Here's the drawing with two shaded views (mm, measured from the low corner). I have some questions. A direction names the side the tool comes from. Round coordinates to 2 decimals unless told otherwise and drop trailing zeros. Loops run counter-clockwise (first coordinate to the right, second up) from the corner with the lowest first, then second, coordinate; pieces in that order, holes last. Notation, with made-up numbers: (65.5, 50.5) -> (115.5, 50.5) arc R20 cw to (115.5, 65.5) -> close; hole circle Ø3 at (-23, 13). An arc over 180 degrees is marked (long way). Use a Markdown table: item, result.
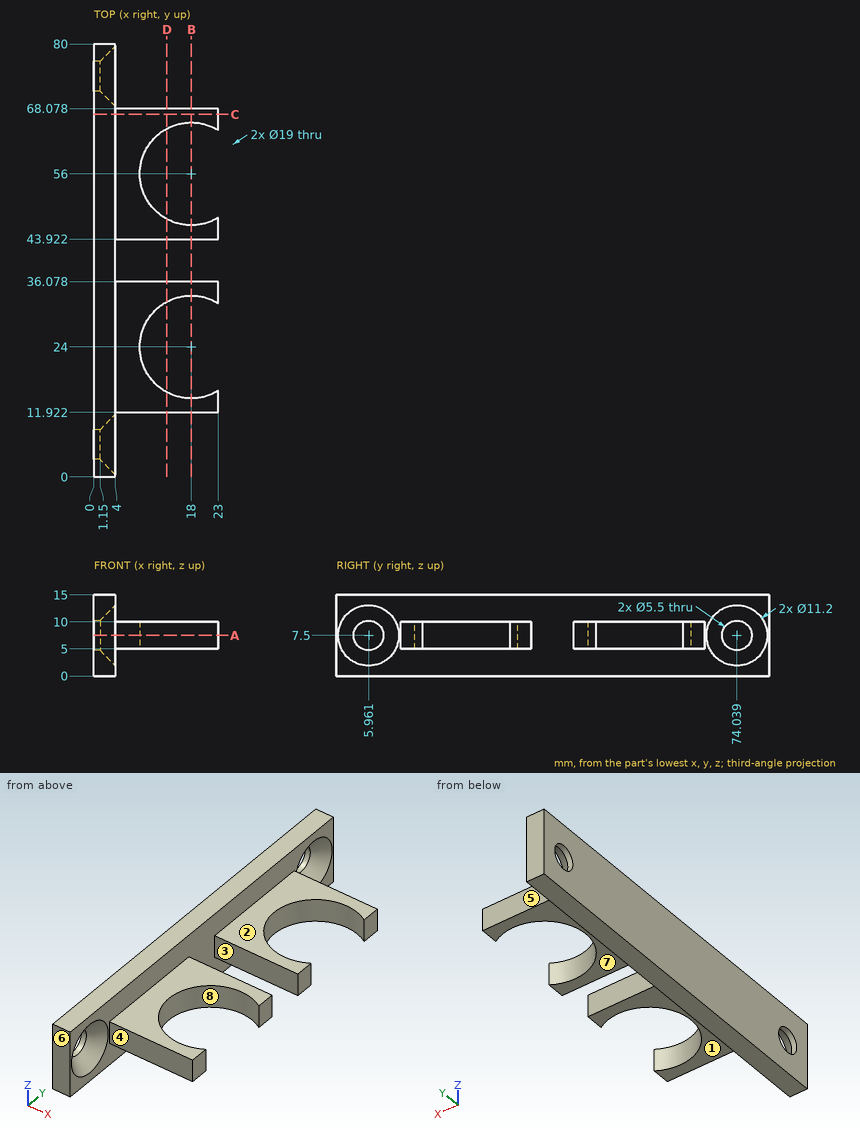
1. I want a section at D-D (x = 13.5). Please give me the cut outline in (y, z).
Answer sheet:
| item | result |
|---|---|
| outline | (11.92, 5) -> (15.63, 5) -> (15.63, 10) -> (11.92, 10) -> close; (32.37, 5) -> (36.08, 5) -> (36.08, 10) -> (32.37, 10) -> close; (43.92, 5) -> (47.63, 5) -> (47.63, 10) -> (43.92, 10) -> close; (64.37, 5) -> (68.08, 5) -> (68.08, 10) -> (64.37, 10) -> close |
2. Which directions (+Z, -Z, +X, -X, +Y, -Y) give clear straight access to the entire face, cutting with the end or side of a thin tool? Please do the marked faces 1, 2, 3, 4 and 5.
Answer sheet:
| item | result |
|---|---|
| face 1 | -Z, +X, +Y, -Y |
| face 2 | +Z, +X, +Y, -Y |
| face 3 | +Z, -Z, +X |
| face 4 | +Z, -Z, +X, -Y |
| face 5 | +Z, -Z, +X, +Y |
3. I want a section at B-B (x = 18). Please give me the cut outline in (y, z).
Answer sheet:
| item | result |
|---|---|
| outline | (11.92, 5) -> (14.5, 5) -> (14.5, 10) -> (11.92, 10) -> close; (33.5, 5) -> (36.08, 5) -> (36.08, 10) -> (33.5, 10) -> close; (43.92, 5) -> (46.5, 5) -> (46.5, 10) -> (43.92, 10) -> close; (65.5, 5) -> (68.08, 5) -> (68.08, 10) -> (65.5, 10) -> close |
4. I need wall thicknesses on line 1 (Y direction, x = 18, z = 6.5); line 2 (Y direction, x = 0.45, z = 7.5); line 3 (Y direction, x = 6.25, z = 8.25). Which ranges of each line are inside material? Lowest first, please.
Answer sheet:
| item | result |
|---|---|
| line 1 | y = 11.92 to 14.5, 33.5 to 36.08, 43.92 to 46.5, 65.5 to 68.08 |
| line 2 | y = 0 to 3.21, 8.71 to 71.29, 76.79 to 80 |
| line 3 | y = 11.92 to 36.08, 43.92 to 68.08 |
5. If we mould it in two halves opening along Y, with no side actions, what happens to the marked faces 6, 7 and 8? For each: +Y half, -Y half, draft (parallel to the pull), parting line (faces both ways), or undercut.
Answer sheet:
| item | result |
|---|---|
| face 6 | -Y half |
| face 7 | draft |
| face 8 | undercut |
6. Will these pins go through, and if not, where does the flat tip stop? pin 1 Ø6 at (y, z) = (38, 12) entering from +X; pin 2 Ø8 at (x, z) = (15.5, 8.5) entering from -Y; pin 3 Ø6 at (x, y) = (10.5, 50.5) entering from -Z; pin 4 Ø9.5 at (x, y) = (14.5, 29.5) entering from +Z.
Answer sheet:
| item | result |
|---|---|
| pin 1 | stops at x = 23 |
| pin 2 | stops at y = 11.92 |
| pin 3 | stops at z = 5 |
| pin 4 | stops at z = 10 |
7. I want a section at C-C (y = 67). Please give me the cut outline in (x, z), plus the area to 3 significant figures.
Answer sheet:
| item | result |
|---|---|
| outline | (0, 0) -> (4, 0) -> (4, 5) -> (23, 5) -> (23, 10) -> (4, 10) -> (4, 15) -> (0, 15) -> close |
| area | 155 mm² |
8. I want a section at A-A (z = 7.5). Please give me the cut outline in (x, y).
Answer sheet:
| item | result |
|---|---|
| outline | (0, 0) -> (4, 0) -> (4, 0.36) -> (1.15, 3.21) -> (0, 3.21) -> close; (0, 8.71) -> (1.15, 8.71) -> (4, 11.56) -> (4, 11.92) -> (23, 11.92) -> (23, 15.92) arc R9.5 cw (long way) to (23, 32.08) -> (23, 36.08) -> (4, 36.08) -> (4, 43.92) -> (23, 43.92) -> (23, 47.92) arc R9.5 cw (long way) to (23, 64.08) -> (23, 68.08) -> (4, 68.08) -> (4, 68.44) -> (1.15, 71.29) -> (0, 71.29) -> close; (0, 76.79) -> (1.15, 76.79) -> (4, 79.64) -> (4, 80) -> (0, 80) -> close |
